from build123d import *

# Parameters (mm, degrees)
F4_D     = 3.3
F4_DEPTH = 18.925
F4_TIP   = 0.9914200214
F5_SIZE  = 1


with BuildPart() as f1:
    # F0 (on Front) → F1 (revolve)
    with BuildSketch(Plane.XZ):
        with BuildLine():
            Line((-17.5953409282, 5.5167464038), (-30.0953409282, 5.5167464038))
            Line((-30.0953409282, 5.5167464038), (-30.0953409282, -4.4832535962))
            Line((-30.0953409282, -4.4832535962), (15.5546590718, -4.4832535962))
            Line((15.5546590718, -4.4832535962), (15.5546590718, 0.0167464038))
            ThreePointArc((15.5546590718, 0.0167464038), (15.7011056812, 0.3702997944), (16.0546590718, 0.5167464038))
            Line((16.0546590718, 0.5167464038), (19.0546590718, 0.5167464038))
            Line((19.0546590718, 0.5167464038), (19.0546590718, 5.5167464038))
            Line((19.0546590718, 5.5167464038), (15.0546590718, 5.5167464038))
            Line((15.0546590718, 5.5167464038), (15.0546590718, 3.7667464038))
            Line((15.0546590718, 3.7667464038), (11.9046590718, 3.7667464038))
            Line((11.9046590718, 3.7667464038), (11.9046590718, 5.5167464038))
            Line((11.9046590718, 5.5167464038), (-0.5953409282, 5.5167464038))
            ThreePointArc((-0.5953409282, 5.5167464038), (-0.9488943188, 5.6631930132), (-1.0953409282, 6.0167464038))
            Line((-1.0953409282, 6.0167464038), (-1.0953409282, 7.1772464038))
            Line((-1.0953409282, 7.1772464038), (-17.0953409282, 7.1772464038))
            Line((-17.0953409282, 7.1772464038), (-17.0953409282, 6.0167464038))
            ThreePointArc((-17.0953409282, 6.0167464038), (-17.2417875376, 5.6631930132), (-17.5953409282, 5.5167464038))
        make_face()
    revolve(axis=Axis((13.2239913882, 0, -44.4832535962), (1, 0, 0)))


with BuildPart() as f1_1:
    # F2: moved
    add(f1.part.moved(Location((0, 0, 44.563))))

    # F4
    with Locations(Plane(origin=(-30.0953409282, 0, 0), x_dir=(0, -1, 0), z_dir=(-1, 0, 0))):
        with Locations((0, 46), (23, 39.8371685741), (39.8371685741, 23), (46, 0), (39.8371685741, -23), (23, -39.8371685741), (0, -46), (-23, -39.8371685741), (-39.8371685741, -23), (-46, 0), (-39.8371685741, 23), (-23, 39.8371685741)):
            Hole(F4_D / 2, depth=F4_DEPTH)
            with Locations((0, 0, -(F4_DEPTH + F4_TIP / 2))):  # 118° drill point
                Cone(0, F4_D / 2, F4_TIP, mode=Mode.SUBTRACT)

    # F5
    f5_edges = [f1_1.edges().sort_by_distance(p)[0] for p in [
        (-30.095341, 0, -39.920254),
        (15.554659, 0, -39.920254),
        (-7.270341, 0, 40.079746),
        (19.054659, 0, -49.920254),
    ]]
    chamfer(f5_edges, length=F5_SIZE)


solid = f1_1.part
Could you check a few things on this model? Use its own coordinates, in mm. A direction names the side the tool comes from. Give positions to 0.01 mm unless a question says otherwise; leave off trailing zeros. Write each loop counter-clockwise with the first axis right and the second up, starting at its lowest first coordinate (ties: lowest second). Pieces come first, ordered by that corner, then holes. Notation, with made-up numbers: (64.25, -25) -> (89.25, -25) arc R29 ccw to (89.25, 8) -> close; hole circle Ø9 at (1, 1.25). An arc over 180 degrees is marked (long way). Answer as CSV lines item,"result". Start each with the question number.
(1) If we section it at C-C, the plane x = -5: Write out the boundary of the cut face in (y, z).
(2) Please list where these lines run through material, in increasing order: line 1 (Y direction, x = -20, z = 23); line 2 (Z direction, x = -3.5, y = 1); line 3 (Y direction, x = -14, z = -40.5).
(3) If we section it at A-A, the plane x = 9: Write out the boundary of the cut face in (y, z), and give its area (3 significant figures).
(4) I'm going to push flat-ended pins straight in: pin 1 Ø6 at (x, z) = (12.5, 25) entering from +Y; pin 2 Ø6 at (x, y) = (12, -39.5) entering from +Z; pin 3 Ø10 at (x, y) = (-18.5, 5) entering from -Z; pin 4 Ø5.5 at (y, z) = (23, 39.84) entering from -X. Where does each tip first touch, or does it pass through?
(5) Which directions (+Z, -Z, +X, -X, +Y, -Y) give clear straight access to the entire face, cutting with the end or side of a thin tool? Please do faces 5 (the face through (-20.5, -24.22, 40.95)), 6 (the face through (-1.095, 50, -11)), 7 (the face through (15.055, -41, -26)).
(6) If we mould it in two halves opening along Z, with no side actions, what happens to faces 1 (the face through (-20.5, -41.486, -22.927)), 2 (the face through (-23.93, 30.42, -39.6)), 3 (the face through (-20.5, 44.35, 0.07)), 4 (the face through (-30.095, 41, -8))? For each: +Z half, -Z half, draft (parallel to the pull), parting line (faces both ways), or undercut.
(7) If we section it at B-B, the plane x = -27: Give the number of separate pieces and of enclosed holes in the cut face, and give its area (3 significant figures).
Answer list:
1,outline,"circle Ø103.32 at (0, 0.08); hole circle Ø80 at (0, 0.08)"
2,line 1,"-44.44 to -41.49, -38.19 to -32.78, 32.78 to 38.19, 41.49 to 44.44"
2,line 2,"-51.57 to -39.91, 40.07 to 51.73"
2,line 3,"-31.97 to -24.51, -21.49 to 21.49, 24.51 to 31.97"
3,outline,"circle Ø100 at (0, 0.08); hole circle Ø80 at (0, 0.08)"
3,area,"2,830 mm^2"
4,pin 1,"y = 44.91"
4,pin 2,"z = 34.25"
4,pin 3,"z = -51.58"
4,pin 4,"x = -30.1"
5,face 5,"-X"
5,face 6,"+X"
5,face 7,"none"
6,face 1,"undercut"
6,face 2,"parting line"
6,face 3,"undercut"
6,face 4,"draft"
7,separate pieces,"1"
7,enclosed holes,"13"
7,area,"2,720 mm^2"
